The drawing under review shows one solid part. Ordinate dimensions are in mm from its lowest x, y, z. A direction names the side the tool comes from. Round coordinates to 2 decimals unless told otherwise and drop trailing zeros. Loops run counter-clockwise (first coordinate to the right, second up) from the corner with the lowest first, then second, coordinate; pieces in that order, holes last. Notation, with made-up numbers: M 2,-21.5 L 38,-21.5 A20 cw 38,1.5 Z; hole C -6.75,62.25 d10. An arc over 180 degrees is marked long. Use a Markdown table: item, result.
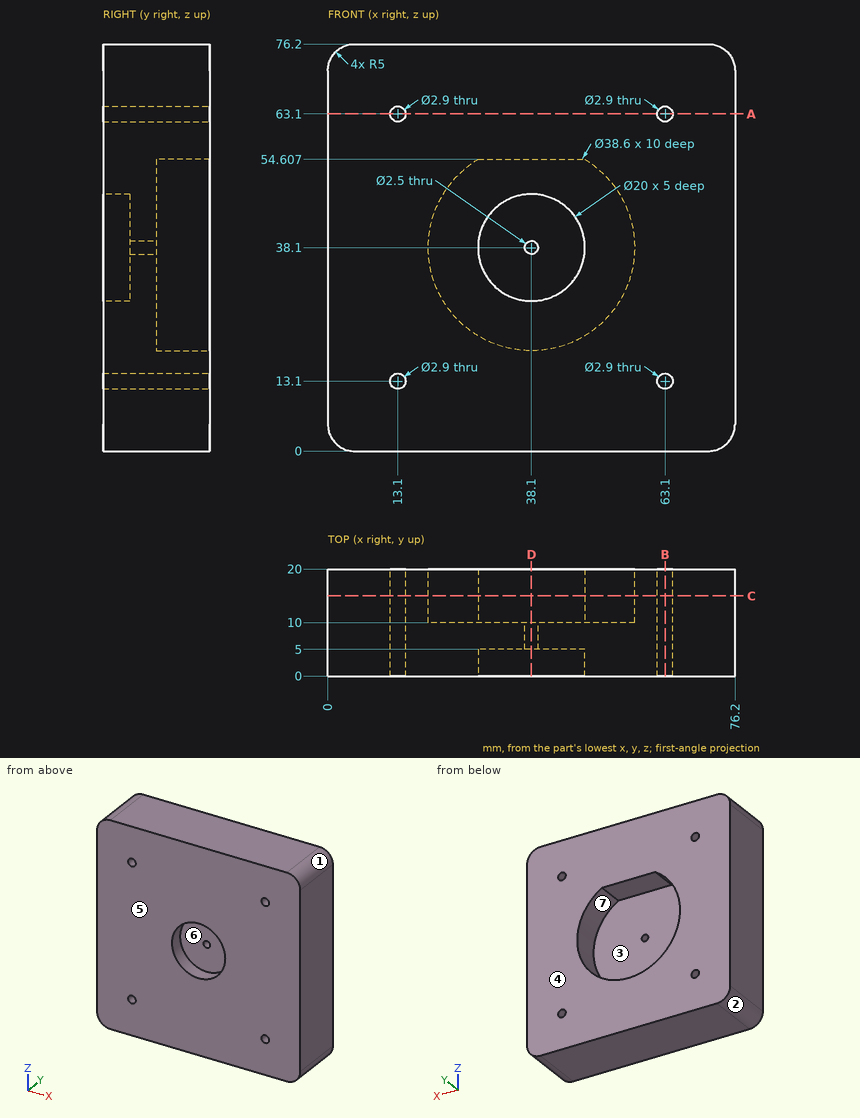
1. Insertion check: pin 1 (16 mm diameter, centred on x = 38.1, z = 38.1, fed in from -Y); pin 2 (3 mm diameter, centred on x = 38.1, z = 38.1, fed in from +Y). Each pin has a flat end and moves straight along its axis. Give the tip position at first contact, or say it passes through.
Check values:
| item | result |
|---|---|
| pin 1 | stops at y = 5 |
| pin 2 | stops at y = 10 |
2. Machinability: for the marked faces 5, 6 and 7, which of the approach directions +Z, -Z, +X, -X, +Y, -Y give a long, thin tool a straight path to every point of the face, cutting with its end or side? Answer none if there is none.
Check values:
| item | result |
|---|---|
| face 5 | +Z, -Z, +X, -X, -Y |
| face 6 | -Y |
| face 7 | +Y |
3. The part is to be moulded in two halves that separate along Z. For the marked faces 1, 2, 3 and 4, say which applies: pulls with the +Z half, pulls with the -Z half, needs draft (parallel to the pull), parting line crosses it, or undercut.
Check values:
| item | result |
|---|---|
| face 1 | pulls with the +Z half |
| face 2 | pulls with the -Z half |
| face 3 | undercut |
| face 4 | needs draft |
4. Take a section at D-D on x = 38.1. Give the boundary of the cut face in (y, z), and give its area (3 significant figures).
Check values:
| item | result |
|---|---|
| outline | M 0,0 L 20,0 L 20,18.8 L 10,18.8 L 10,36.85 L 5,36.85 L 5,28.1 L 0,28.1 Z; M 0,48.1 L 5,48.1 L 5,39.35 L 10,39.35 L 10,54.61 L 20,54.61 L 20,76.2 L 0,76.2 Z |
| area | 1,050 mm² |
5. Take a section at C-C on y = 15. Give the boundary of the cut face in (x, z), and give its area (3 significant figures).
Check values:
| item | result |
|---|---|
| outline | M 0,5 A5 ccw 5,0 L 71.2,0 A5 ccw 76.2,5 L 76.2,71.2 A5 ccw 71.2,76.2 L 5,76.2 A5 ccw 0,71.2 Z; hole C 13.1,13.1 d2.9; hole C 13.1,63.1 d2.9; hole M 28.1,54.61 A19.3 ccw long 48.1,54.61 Z; hole C 63.1,13.1 d2.9; hole C 63.1,63.1 d2.9 |
| area | 4,630 mm² |
6. Take a section at A-A on z = 63.1. Give the boundary of the cut face in (x, y), and give its area (3 significant figures).
Check values:
| item | result |
|---|---|
| outline | M 0,0 L 11.65,0 L 11.65,20 L 0,20 Z; M 14.55,0 L 61.65,0 L 61.65,20 L 14.55,20 Z; M 64.55,0 L 76.2,0 L 76.2,20 L 64.55,20 Z |
| area | 1,410 mm² |
7. Take a section at B-B on x = 63.1. Give the boundary of the cut face in (y, z), and give its area (3 significant figures).
Check values:
| item | result |
|---|---|
| outline | M 0,0 L 20,0 L 20,11.65 L 0,11.65 Z; M 0,14.55 L 20,14.55 L 20,61.65 L 0,61.65 Z; M 0,64.55 L 20,64.55 L 20,76.2 L 0,76.2 Z |
| area | 1,410 mm² |
8. Wall thickness on line 1 along Z through (x, y) = (63.1, 11.75); line 2 along X through (y, z) = (8.05, 38.1): over which ranges is each line inside the solid? List them lowest first. Write a range as from..to.
Check values:
| item | result |
|---|---|
| line 1 | z = 0..11.65, 14.55..61.65, 64.55..76.2 |
| line 2 | x = 0..36.85, 39.35..76.2 |
